from build123d import *

# Parameters (mm, degrees)
SZKIC1_W                    = 275
SZKIC1_H                    = 50
DODANIE_WYCI_GNI_CIE1_DEPTH = 5
SZKIC2_W                    = 35
SZKIC2_H                    = 35
SZKIC2_R                    = 7
DODANIE_WYCI_GNI_CIE2_DEPTH = 5


with BuildPart() as part:
    # Szkic1 → Dodanie-wyciągnięcie1 (new body)
    with BuildSketch(Plane(origin=(0, 0, 0), x_dir=(1, 0, 0), z_dir=(0, 1, 0))):
        with Locations((137.5, 25)):
            Rectangle(SZKIC1_W, SZKIC1_H)
    extrude(amount=DODANIE_WYCI_GNI_CIE1_DEPTH)

    # Szkic2 → Dodanie-wyciągnięcie2 (add)
    with BuildSketch(Plane.XY):
        with Locations((17.5, 17.5)):
            Rectangle(SZKIC2_W, SZKIC2_H)
        with Locations((17.5, 22.5)):
            Circle(SZKIC2_R, mode=Mode.SUBTRACT)
        with Locations((257.5, 17.5)):
            Rectangle(SZKIC2_W, SZKIC2_H)
        with Locations((257.5, 22.5)):
            Circle(SZKIC2_R, mode=Mode.SUBTRACT)
    dodanie_wyci_gni_cie2 = extrude(amount=DODANIE_WYCI_GNI_CIE2_DEPTH)

    # Lustro1: Dodanie-wyciągnięcie2 across plane
    add(dodanie_wyci_gni_cie2.mirror(Plane(origin=(0, 0, -25), x_dir=(1, 0, 0), z_dir=(0, 0, -1))))


solid = part.part
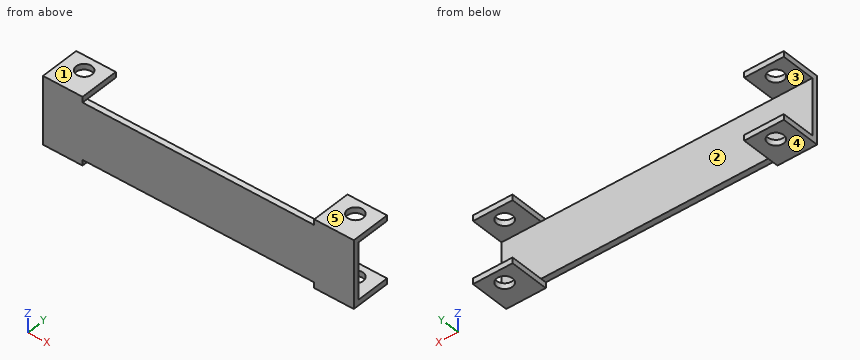
Work out the finished part from the listing and answer in its coordinate system (mm). Face numbers are marked on the shaded views. A direction names the side the tool comes from. Give positions to 0.01 mm unless a question says otherwise; leave off trailing zeros. Loops run counter-clockwise (first coordinate to the right, second up) from the corner with the lowest first, then second, coordinate; pieces in that order, holes last. Notation, with made-up numbers: (-29.5, 19) -> (-1.5, 19) arc R27 ccw to (-1.5, 40) -> close; hole circle Ø3 at (56, 30). An arc over 180 degrees is marked (long way). Use a Markdown table: item, result. Add a question column.
1. Section B-B on y = 22.5 is taken. State how many separate pieces and enclosed holes the cut face has, and give its area (3 significant figures).
2. Find the intervals of material crossed by probe 1 along X at (y, z) = (22, -51); probe 2 along Y at (x, z) = (17.5, 2.7); probe 3 along X at (y, z) = (13.5, 2), in increasing order.
3. Section C-C on y = 8 is taken. Determine the outline of the cut face in (x, z), and give its area (3 significant figures).
4. Section A-A on x = 257.5 is taken. Determine the outline of the cut face in (y, z), and give its area (3 significant figures).
5. Determine the mould class of the marked faces 3, 4 and 5 for opening direction Z: released by +Z, released by -Z, zero draft, split by the parting line, or undercut.
6. Flat-ended cylindrical pins translate along their axes: pin 1 Ø4 at (x, y) = (126, 3.5) entering from -Z; pin 2 Ø1 at (x, z) = (194.5, -20.5) entering from +Y; pin 3 Ø2.5 at (x, y) = (187, 2.5) entering from +Z. Find the tip coordinate at first contact, or state that the pin passes through.
7. For the marked faces 1 and 2, determine the directions among +Z, -Z, +X, -X, +Y, -Y from which every point of the face is accessible in a straight line to the end or side of a thin tool.
8. Section D-D on z = -35 is taken. Determine the outline of the cut face in (x, y), and give its area (4 significant figures).
Results below:
| question | item | result |
|---|---|---|
| 1 | separate pieces | 8 |
| 1 | enclosed holes | 0 |
| 1 | area | 420 mm^2 |
| 2 | probe 1 | x = 0 to 10.52, 24.48 to 35, 240 to 250.52, 264.48 to 275 |
| 2 | probe 2 | y = 0 to 15.5, 29.5 to 35 |
| 2 | probe 3 | x = 0 to 35, 240 to 275 |
| 3 | outline | (0, -55) -> (35, -55) -> (35, -50) -> (0, -50) -> close; (0, 0) -> (35, 0) -> (35, 5) -> (0, 5) -> close; (240, -55) -> (275, -55) -> (275, -50) -> (240, -50) -> close; (240, 0) -> (275, 0) -> (275, 5) -> (240, 5) -> close |
| 3 | area | 700 mm^2 |
| 4 | outline | (0, -55) -> (15.5, -55) -> (15.5, -50) -> (5, -50) -> (5, 0) -> (15.5, 0) -> (15.5, 5) -> (0, 5) -> close; (29.5, -55) -> (35, -55) -> (35, -50) -> (29.5, -50) -> close; (29.5, 0) -> (35, 0) -> (35, 5) -> (29.5, 5) -> close |
| 4 | area | 460 mm^2 |
| 5 | face 3 | undercut |
| 5 | face 4 | released by -Z |
| 5 | face 5 | released by +Z |
| 6 | pin 1 | stops at z = -50 |
| 6 | pin 2 | stops at y = 5 |
| 6 | pin 3 | stops at z = 0 |
| 7 | face 1 | +Z, +X, -X, +Y, -Y |
| 7 | face 2 | +X, -X, +Y |
| 8 | outline | (0, 0) -> (275, 0) -> (275, 5) -> (0, 5) -> close |
| 8 | area | 1,375 mm^2 |
